Input: part model. Units: mm. Frame: model coordinates. A direction names the side the tool comes from. Coordinates: 2 decimals unless noted, no trailing zeros. Write each loop counter-clockwise with the first axis right and the second up, starting at its lowest first coordinate (ties: lowest second). Pieces come first, ordered by that corner, then holes. Notation, with made-up numbers: M 84,-24.5 L 107,-24.5 A9 ccw 107,-18.5 Z; hole C -34.75,26 d10. An arc over 180 degrees is marked long. Use one line per item in the form item = value.
from build123d import *

# Parameters (mm, degrees)
F0_R     = 6
F1_DEPTH = 1.5
F2_R     = 3.95
F3_DEPTH = 3
F5_D     = 3


with BuildPart() as f1:
    # F0 (on Front) → F1 (new body)
    with BuildSketch(Plane.XZ):
        Circle(F0_R)
    extrude(amount=F1_DEPTH)

    # F2 (on face) → F3 (join)
    with BuildSketch(Plane.XZ.offset(1.5)):
        Circle(F2_R)
    extrude(amount=F3_DEPTH)

    # F5 (through all)
    with Locations(Plane.XZ.offset(4.5)):
        with Locations((0, 0)):
            Hole(F5_D / 2)


solid = f1.part
(1) Section query B-B on x = 0. Return the cut outline in (y, z).
Computed:
outline = M -4.5,-3.95 L -1.5,-3.95 L -1.5,-6 L 0,-6 L 0,-1.5 L -4.5,-1.5 Z; M -4.5,1.5 L 0,1.5 L 0,6 L -1.5,6 L -1.5,3.95 L -4.5,3.95 Z
(2) Section query C-C on y = -2.15. Return the cut outline in (x, z), plus the area to 3 significant figures.
Computed:
outline = C 0,0 d7.9; hole C 0,0 d3
area = 41.9 mm^2
(3) First-contact query: pin 1 Ø3.5 at (x, z) = (1, 0.5) entering from -Y; pin 2 Ø4 at (x, z) = (-4.5, 4.5) entering from -Y. Flat tips, straight axial feed; report the tip coordinate or a pass-through.
Computed:
pin_1 = -4.5
pin_2 = -1.5
(4) Pull-direction query (Z, two-part tool) for faces 1 (the flat face through (1.2, 0, -1.2)), 2 (the cylindrical face through (-3.135, -2.979, -2.404)), 3 (the cylindrical face through (1.5, -2.22, 0.07)); classes: pulls with the +Z half, pulls with the -Z half, needs draft (parallel to the pull), parting line crosses it, or undercut.
Computed:
face_1 = needs draft
face_2 = parting line crosses it
face_3 = undercut
(5) Set-up query: faces 4 (the flat face through (1, -1.5, -4)), 5 (the flat face through (2, -4.5, 0)). Return all of +Z, -Z, +X, -X, +Y, -Y with unobstructed straight access to the full face (end or side cutting, diameter ignored); none if empty.
Computed:
face_4 = -Y
face_5 = +Z, -Z, +X, -X, -Y
(6) Section query D-D on x = 1.75. Return the cut outline in (y, z), plus the area to 3 significant figures.
Computed:
outline = M -4.5,-3.54 L -1.5,-3.54 L -1.5,-5.74 L 0,-5.74 L 0,5.74 L -1.5,5.74 L -1.5,3.54 L -4.5,3.54 Z
area = 38.5 mm^2
(7) Section query A-A on z = 0. Return the cut outline in (x, y).
Computed:
outline = M -6,-1.5 L -3.95,-1.5 L -3.95,-4.5 L -1.5,-4.5 L -1.5,0 L -6,0 Z; M 1.5,-4.5 L 3.95,-4.5 L 3.95,-1.5 L 6,-1.5 L 6,0 L 1.5,0 Z
(8) Line query: probe 1 along Z at (x, y) = (0, -3.25); probe 2 along Z at (x, y) = (0, -1.4); probe 3 along Y at (x, z) = (1.25, 4.75). Output: solid intervals per line, ascending.
Computed:
probe_1 = -3.95 to -1.5, 1.5 to 3.95
probe_2 = -6 to -1.5, 1.5 to 6
probe_3 = -1.5 to 0
